Can you work these out from the model? Positions are in its coordinate system, mm. Face numbers are marked on the shaded views. A direction names the side the tool comes from. Round coordinates to 2 decimals unless told otherwise and drop trailing zeros. Order: outer loops, then holes, each group sorted by start corner. A loop starts at its lowest first (then second) coordinate and runs counter-clockwise, first axis right, second up. Notation, with made-up numbers: M 38.5,47 L 71.5,47 A15 cw 71.5,74 Z; hole C -5.75,86.25 d8. An arc over 180 degrees is marked long. One line per question, with ' | ' between items.
```python
from build123d import *

# Parameters (mm, degrees)
SKETCH1_W           = 70
SKETCH1_H           = 50
BOSS_EXTRUDE1_DEPTH = 50
CUT_EXTRUDE1_DEPTH  = 50
SKETCH3_W           = 40
SKETCH3_H           = 10
CUT_EXTRUDE2_DEPTH  = 50
CUT_EXTRUDE3_DEPTH  = 30
BOSS_EXTRUDE2_DEPTH = 30
SKETCH9_W           = 20
SKETCH9_H           = 10
BOSS_EXTRUDE3_DEPTH = 5
CUT_EXTRUDE5_DEPTH  = 5
SKETCH15_W          = 70
SKETCH15_H          = 50
CUT_EXTRUDE10_DEPTH = 19
CUT_EXTRUDE11_DEPTH = 19
SKETCH18_W          = 67.082039325
SKETCH18_H          = 30
BOSS_EXTRUDE8_DEPTH = 10
SKETCH19_W          = 50
SKETCH19_H          = 20
CUT_EXTRUDE12_DEPTH = 10
SKETCH20_W          = 45
SKETCH20_H          = 76.778692576
CUT_EXTRUDE13_DEPTH = 28
CUT_EXTRUDE14_DEPTH = 28
SKETCH22_W          = 20
SKETCH22_H          = 10
CUT_EXTRUDE15_DEPTH = 30
CUT_EXTRUDE16_DEPTH = 10
CUT_EXTRUDE17_DEPTH = 10
CUT_EXTRUDE18_DEPTH = 10
CUT_EXTRUDE19_DEPTH = 5


with BuildPart() as part:
    # Sketch1 → Boss-Extrude1 (new body)
    with BuildSketch(Plane.XY):
        with Locations((35, 25)):
            Rectangle(SKETCH1_W, SKETCH1_H)
    extrude(amount=BOSS_EXTRUDE1_DEPTH)

    # Sketch2 → Cut-Extrude1 (cut)
    with BuildSketch(Plane.XY.offset(50)):
        Polygon((0, 50), (60, 50), (0, 20), align=None)
    extrude(amount=-CUT_EXTRUDE1_DEPTH, mode=Mode.SUBTRACT)

    # Sketch3 → Cut-Extrude2 (cut)
    with BuildSketch(Plane(origin=(70, 0, 0), x_dir=(0, 0, -1), z_dir=(1, 0, 0))):
        with Locations((-30, 45)):
            Rectangle(SKETCH3_W, SKETCH3_H)
    extrude(amount=-CUT_EXTRUDE2_DEPTH, mode=Mode.SUBTRACT)

    # Sketch4 → Cut-Extrude3 (cut)
    with BuildSketch(Plane.XY.offset(50)):
        Polygon((60, 10), (60, 40), (40, 40), (0, 20), (0, 10), align=None)
    extrude(amount=-CUT_EXTRUDE3_DEPTH, mode=Mode.SUBTRACT)

    # Sketch8 → Boss-Extrude2 (add)
    with BuildSketch(Plane(origin=(-8, 16, 0), x_dir=(0.894427191, 0.447213595, 0), z_dir=(-0.447213595, 0.894427191, 0))):
        Polygon((8.94427191, -20), (8.94427191, -40), (53.66563146, -20), align=None)
    extrude(amount=-BOSS_EXTRUDE2_DEPTH)

    # Sketch9 → Boss-Extrude3 (add)
    with BuildSketch(Plane.ZY):
        with Locations((30, 15)):
            Rectangle(SKETCH9_W, SKETCH9_H)
    extrude(amount=-BOSS_EXTRUDE3_DEPTH)

    # Sketch10 → Cut-Extrude5 (cut)
    with BuildSketch(Plane.XZ):
        Polygon((10, 40), (27.082039325, 33.16718427), (27.082039325, 20), (10, 20), align=None)
    extrude(amount=CUT_EXTRUDE5_DEPTH, mode=Mode.SUBTRACT)

    # Sketch15 → Cut-Extrude10 (cut)
    with BuildSketch(Plane(origin=(0, 0, 0), x_dir=(-1, 0, 0), z_dir=(0, -1, 0))):
        with Locations((-35, -25)):
            Rectangle(SKETCH15_W, SKETCH15_H)
    extrude(amount=CUT_EXTRUDE10_DEPTH, mode=Mode.SUBTRACT)

    # Sketch16 → Cut-Extrude11 (cut)
    with BuildSketch(Plane(origin=(14.666666667, 7.333333333, 36.666666667), x_dir=(0.930949336, -0.071611487, -0.358057437), z_dir=(0.365148372, 0.182574186, 0.912870929))):
        Polygon((-15.754527229, 11.766968108), (-10.383665674, 12.159200379), (-10.383665674, 1.961161351), (-16.527761833, 3.611754734), align=None)
    extrude(amount=CUT_EXTRUDE11_DEPTH, mode=Mode.SUBTRACT)

    # Sketch18 → Boss-Extrude8 (add)
    with BuildSketch(Plane(origin=(20, 0, 40), x_dir=(0.894427191, 0, -0.447213595), z_dir=(0.447213595, 0, 0.894427191))):
        with Locations((11.180339888, 25)):
            Rectangle(SKETCH18_W, SKETCH18_H)
    extrude(amount=-BOSS_EXTRUDE8_DEPTH)

    # Sketch19 → Cut-Extrude12 (cut)
    with BuildSketch(Plane.ZY):
        with Locations((25, 10)):
            Rectangle(SKETCH19_W, SKETCH19_H)
    extrude(amount=CUT_EXTRUDE12_DEPTH, mode=Mode.SUBTRACT)

    # Sketch20 → Cut-Extrude13 (cut)
    with BuildSketch(Plane(origin=(-8, 16, 0), x_dir=(0.894427191, 0.447213595, 0), z_dir=(-0.447213595, 0.894427191, 0))):
        with Locations((31.44427191, -38.389346288)):
            Rectangle(SKETCH20_W, SKETCH20_H)
    extrude(amount=CUT_EXTRUDE13_DEPTH, mode=Mode.SUBTRACT)

    # Sketch21 → Cut-Extrude14 (cut)
    with BuildSketch(Plane(origin=(8, 4, 0), x_dir=(0, 0, -1), z_dir=(0.894427191, 0.447213595, 0))):
        Polygon((-50, 17.88854382), (-38.819660113, 17.88854382), (-41.05572809, 27.88854382), align=None)
    extrude(amount=-CUT_EXTRUDE14_DEPTH, mode=Mode.SUBTRACT)

    # Sketch22 → Cut-Extrude15 (cut)
    with BuildSketch(Plane(origin=(0, 40, 0), x_dir=(1, 0, 0), z_dir=(0, 1, 0))):
        with Locations((50, -25)):
            Rectangle(SKETCH22_W, SKETCH22_H)
    extrude(amount=-CUT_EXTRUDE15_DEPTH, mode=Mode.SUBTRACT)

    # Sketch23 → Cut-Extrude16 (cut)
    with BuildSketch(Plane(origin=(24, 0, 32), x_dir=(0.8, 0, -0.6), z_dir=(0.6, 0, 0.8))):
        Polygon((20, 40), (-30, 20), (-30, 10), (20, 10), align=None)
    extrude(amount=CUT_EXTRUDE16_DEPTH, mode=Mode.SUBTRACT)

    # Sketch24 → Cut-Extrude17 (cut)
    with BuildSketch(Plane(origin=(-8.827586207, 27.586206897, 6.620689655), x_dir=(0.954842468, 0.288908462, 0.069338031), z_dir=(0.297112541, -0.928476691, -0.222834406))):
        Polygon((51.136797811, 10.112827941), (51.136797811, 20.396796046), (9.245070791, 43.95190605), align=None)
    extrude(amount=-CUT_EXTRUDE17_DEPTH, mode=Mode.SUBTRACT)

    # Sketch25 → Cut-Extrude18 (cut)
    with BuildSketch(Plane(origin=(40, 0, 0), x_dir=(0, 0, -1), z_dir=(1, 0, 0))):
        Polygon((-30, 40), (-20, 40), (-30, 37.6), align=None)
    extrude(amount=-CUT_EXTRUDE18_DEPTH, mode=Mode.SUBTRACT)

    # Sketch26 → Cut-Extrude19 (cut)
    with BuildSketch(Plane(origin=(20, 0, 40), x_dir=(0.894427191, 0, -0.447213595), z_dir=(0.447213595, 0, 0.894427191))):
        Polygon((21.632516526, 39.674355495), (22.360679775, 40), (22.360679775, 37.6), align=None)
    extrude(amount=-CUT_EXTRUDE19_DEPTH, mode=Mode.SUBTRACT)


solid = part.part
```
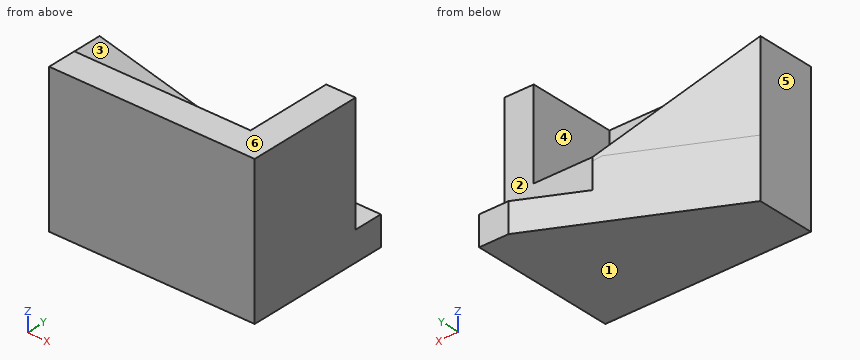
(1) If we section it at C-C on y = 23.5: Please give me the cut outline in (x, z), plus the area to 3 significant figures.
Final values:
outline: M 7,0 L 70,0 L 70,50 L 60,50 L 60,20 L 40,20 L 7,44.75 Z | area: 1,970 mm^2
(2) If we section it at D-D on z = 9: Please give me the cut outline in (x, y), plus the area to 3 significant figures.
Final values:
outline: M 0,0 L 70,0 L 70,50 L 60,50 L 0,20 Z | area: 2,600 mm^2
(3) On a 3-axis mill with a long thin cutter (end or side, diameter ignored), from which of +Z, -Z, +X, -X, +Y, -Y can I reach the whole of each face in a straight line? I mean the marked faces 1, 2 and 3. Say none if no direction works.
Final values:
face 1: -Z, +X, -X, +Y, -Y | face 2: +Z, +X, -X, +Y | face 3: +Z, +Y
(4) Thinking about a two-plate mould opening in X: for the marked faces 4, 5 and 6, which applies, released by +X, released by -X, zero draft, split by the parting line, or undercut?
Final values:
face 4: undercut | face 5: released by -X | face 6: zero draft
(5) Please list where these lines run through material, in increasing order: probe 1 along Y at (x, z) = (51.5, 30.5); probe 2 along X at (y, z) = (29.5, 46.5); probe 3 along X at (y, z) = (20, 28). Write a range as [from, to].
Final values:
probe 1: [0, 10] | probe 2: [60, 70] | probe 3: [0, 29.33], [60, 70]
(6) If we section it at B-B on x = 27: Please give me the cut outline in (y, z).
Final values:
outline: M 0,0 L 33.5,0 L 33.5,29.75 L 10,29.75 L 10,50 L 0,50 Z
(7) If we section it at A-A on z = 35: Please give me the cut outline in (x, y), plus the area to 3 significant figures.
Final values:
outline: M 0,0 L 70,0 L 70,40 L 60,40 L 60,10 L 20,10 L 20,30 L 0,20 Z | area: 1,300 mm^2
(8) Will these pins go through, and if not, where does the flat tip stop? pin 1 Ø6 at (x, y) = (47.5, 18) entering from +Z; pin 2 Ø9 at (y, z) = (31.5, 36.5) entering from -X; pin 3 Ø9 at (x, z) = (21.5, 40.5) entering from +Y.
Final values:
pin 1: z = 20 | pin 2: x = 14 | pin 3: y = 10
